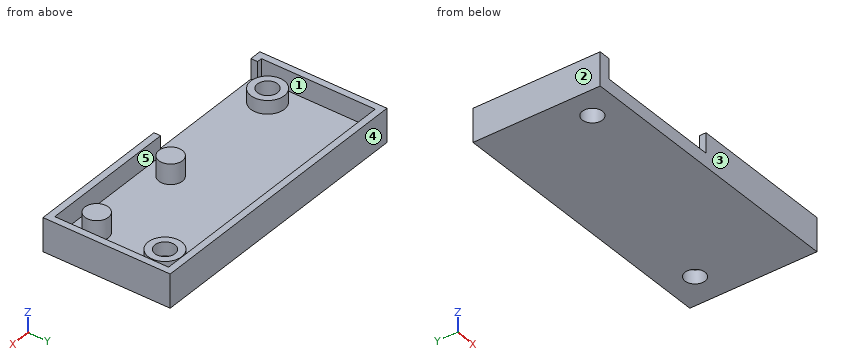
```python
from build123d import *

# Parameters (mm, degrees)
SKETCH001_W   = 42.5
SKETCH001_H   = 19
SKETCH001_W_2 = 40.5
SKETCH001_H_2 = 17
PAD_DEPTH     = 3
SKETCH002_W   = 42.5
SKETCH002_H   = 19
SKETCH002_R   = 1.5
PAD001_DEPTH  = 2
SKETCH003_R   = 1.75
PAD002_DEPTH  = 3
POCKET_DEPTH  = 3.001
SKETCH005_R   = 2.5
SKETCH005_R_2 = 1.5
PAD003_DEPTH  = 2


with BuildPart() as part:
    # Sketch001 → Pad (new body)
    with BuildSketch(Plane.XY):
        with Locations((20, 8.1)):
            Rectangle(SKETCH001_W, SKETCH001_H)
        with Locations((20, 8.1)):
            Rectangle(SKETCH001_W_2, SKETCH001_H_2, mode=Mode.SUBTRACT)
    extrude(amount=PAD_DEPTH)

    # Sketch002 → Pad001 (join)
    with BuildSketch(Plane.XY):
        with Locations((20, 8.1)):
            Rectangle(SKETCH002_W, SKETCH002_H)
        with Locations((3, 3)):
            Circle(SKETCH002_R, mode=Mode.SUBTRACT)
        with Locations((36.5, 13.2)):
            Circle(SKETCH002_R, mode=Mode.SUBTRACT)
    extrude(amount=-PAD001_DEPTH)

    # Sketch003 → Pad002 (join)
    with BuildSketch(Plane.XY):
        with Locations((22, 3)):
            Circle(SKETCH003_R)
        with Locations((36.5, 3)):
            Circle(SKETCH003_R)
    extrude(amount=PAD002_DEPTH)

    # Sketch004 → Pocket (cut, through all)
    with BuildSketch(Plane.XY):
        Polygon((19.5, 0), (5.5, 0), (0.5, 0), (0.5, -1.4), (5.5, -1.4), (19.5, -1.4), align=None)
    extrude(amount=POCKET_DEPTH, mode=Mode.SUBTRACT)

    # Sketch005 → Pad003 (join)
    with BuildSketch(Plane.XY):
        with Locations((3, 3)):
            Circle(SKETCH005_R)
        with Locations((3, 3)):
            Circle(SKETCH005_R_2, mode=Mode.SUBTRACT)
        with Locations((36.5, 13.2)):
            Circle(SKETCH005_R)
        with Locations((36.5, 13.2)):
            Circle(SKETCH005_R_2, mode=Mode.SUBTRACT)
    extrude(amount=PAD003_DEPTH)


solid = part.part
```
The model under review builds one solid part; all positions refer to its coordinate system, in mm. Face numbers are marked on the shaded views. A direction names the side the tool comes from. Round coordinates to 2 decimals unless told otherwise and drop trailing zeros. Loops run counter-clockwise (first coordinate to the right, second up) from the corner with the lowest first, then second, coordinate; pieces in that order, holes last. Notation, with made-up numbers: (-16.5, -6.5) -> (6.5, -6.5) arc R8 cw to (6.5, -2.5) -> close; hole circle Ø11 at (-1.5, 40.5). An arc over 180 degrees is marked (long way). Answer as a JSON object with one key per item and string values. Group by question number.
1) For pin 1 Ø3 at (x, y) = (21.5, 9) entering from +Z; pin 2 Ø5 at (x, y) = (36.5, 13.2) entering from -Z; pin 3 Ø8 at (x, y) = (9, 2) entering from +Z, all flat-tipped, find the tip position at first contact; note any pin that passes through.
2) For the marked faces 1 and 2, list the 3-axis set-ups (+Z, -Z, +X, -X, +Y, -Y) from which the entire face can be reached by the end or side of a thin tool; tool diameter is ignored.
3) We need section C-C on z = 1.45. Write out the cut boundary in (x, y).
4) We need section A-A on y = 13.2. Write out the cut boundary in (x, z), then the cut area to 3 significant figures.
5) We need section B-B on x = 3. Write out the cut boundary in (y, z), then the cut area to 3 significant figures.
6) For line 1 (Y direction, x = 3, z = 0.7); line 2 (Y direction, x = 36.5, z = -1.05); line 3 (Y direction, x = 30, z = 2.2), list the stretches that pass through material, from the lowest coordinate up. Write a range as [from, to].
7) We need section D-D on x = 27. Write out the cut boundary in (y, z), then the cut area to 3 significant figures.
8) Mouldability with a two-part tool opening along Y and no side actions: class the marked faces 3, 4 and 5 as released by +Y, released by -Y, zero draft, split by the parting line, or undercut.
Result set:
{
 "1": {"pin 1": "z = 0", "pin 2": "z = -2", "pin 3": "z = 2"},
 "2": {"face 1": "+Z", "face 2": "+Z, -Z, -X, +Y, -Y"},
 "3": {"outline": "(-1.25, -1.4) -> (0.5, -1.4) -> (0.5, -0.4) -> (-0.25, -0.4) -> (-0.25, 16.6) -> (40.25, 16.6) -> (40.25, -0.4) -> (19.5, -0.4) -> (19.5, -1.4) -> (41.25, -1.4) -> (41.25, 17.6) -> (-1.25, 17.6) -> close; circle Ø5 at (3, 3); circle Ø3.5 at (22, 3); circle Ø5 at (36.5, 13.2); circle Ø3.5 at (36.5, 3); hole circle Ø3 at (3, 3); hole circle Ø3 at (36.5, 13.2)"},
 "4": {"outline": "(-1.25, -2) -> (35, -2) -> (35, 2) -> (34, 2) -> (34, 0) -> (-0.25, 0) -> (-0.25, 3) -> (-1.25, 3) -> close; (38, -2) -> (41.25, -2) -> (41.25, 3) -> (40.25, 3) -> (40.25, 0) -> (39, 0) -> (39, 2) -> (38, 2) -> close", "area": "89.0 mm²"},
 "5": {"outline": "(-1.4, -2) -> (1.5, -2) -> (1.5, 2) -> (0.5, 2) -> (0.5, 0) -> (-1.4, 0) -> close; (4.5, -2) -> (17.6, -2) -> (17.6, 3) -> (16.6, 3) -> (16.6, 0) -> (5.5, 0) -> (5.5, 2) -> (4.5, 2) -> close", "area": "39.0 mm²"},
 "6": {"line 1": "[0.5, 1.5], [4.5, 5.5], [16.6, 17.6]", "line 2": "[-1.4, 11.7], [14.7, 17.6]", "line 3": "[-1.4, -0.4], [16.6, 17.6]"},
 "7": {"outline": "(-1.4, -2) -> (17.6, -2) -> (17.6, 3) -> (16.6, 3) -> (16.6, 0) -> (-0.4, 0) -> (-0.4, 3) -> (-1.4, 3) -> close", "area": "44.0 mm²"},
 "8": {"face 3": "released by -Y", "face 4": "released by +Y", "face 5": "undercut"}
}
